Source: three-view drawing plus pictorial views. Frame: mm from the lowest corner of the part. A direction names the side the tool comes from. Give positions to 0.01 mm unless a question says otherwise; leave off trailing zeros. Order: outer loops, then holes, each group sorted by start corner. A loop starts at its lowest first (then second) coordinate and runs counter-clockwise, first axis right, second up.
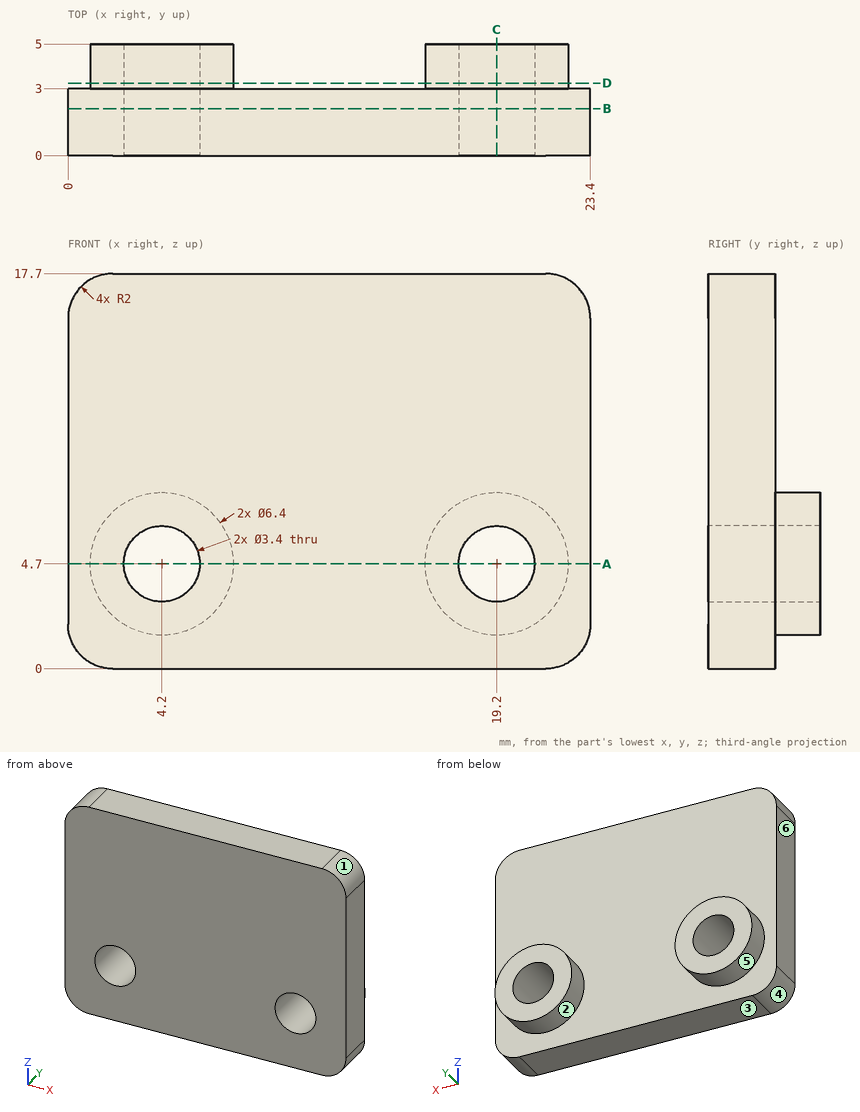
(1) Section A-A, the plane z = 4.7. Return loops of the section in (x, y), plus the area to 3 significant figures.
(2) Section B-B, the plane y = 2.1. Return loops of the section in (x, z).
(3) Section C-C, the plane x = 19.2. Return loops of the section in (y, z).
(4) Draft query along X for the marked faces 1, 2, 3 and 4. Return one class per face: +X half, -X half, draft (parallel to the pull), parting line (faces both ways), or undercut.
(5) Access query for the marked faces 5 and 6. Directions: +Z, -Z, +X, -X, +Y, -Y. A direction counts if a zero-diameter tool reaches every point of the face in a straight line with its end or side. Return the directions, or none.
(6) Line query: line 1 along X through (y, z) = (1.65, 4.7); line 2 along X through (y, z) = (4.3, 3.75); line 3 along X through (y, z) = (3.6, 4.7). Output: solid intervals per line, ascending.
(7) Section D-D, the plane y = 3.25. Return loops of the section in (x, z).
(8) Pin query (flat end, axial travel): pin 1 Ø1.5 at (x, y) = (3.5, 4.5) entering from -Z. Return the tip coordinate at first contact, or that it passes through.
Checks:
1. outline: (0, 0) - (2.5, 0) - (2.5, 5) - (1, 5) - (1, 3) - (0, 3) - close; (5.9, 0) - (17.5, 0) - (17.5, 5) - (16, 5) - (16, 3) - (7.4, 3) - (7.4, 5) - (5.9, 5) - close; (20.9, 0) - (23.4, 0) - (23.4, 3) - (22.4, 3) - (22.4, 5) - (20.9, 5) - close
1. area: 61.8 mm2
2. outline: (0, 2) arc R2 ccw to (2, 0) - (21.4, 0) arc R2 ccw to (23.4, 2) - (23.4, 15.7) arc R2 ccw to (21.4, 17.7) - (2, 17.7) arc R2 ccw to (0, 15.7) - close; hole circle Ø3.4 at (4.2, 4.7); hole circle Ø3.4 at (19.2, 4.7)
3. outline: (0, 0) - (3, 0) - (3, 1.5) - (5, 1.5) - (5, 3) - (0, 3) - close; (0, 6.4) - (5, 6.4) - (5, 7.9) - (3, 7.9) - (3, 17.7) - (0, 17.7) - close
4. face 1: +X half
4. face 2: undercut
4. face 3: draft
4. face 4: -X half
5. face 5: +Y
5. face 6: +Z, -Z, -X, +Y, -Y
6. line 1: x = 0 to 2.5, 5.9 to 17.5, 20.9 to 23.4
6. line 2: x = 1.14 to 2.79, 5.61 to 7.26, 16.14 to 17.79, 20.61 to 22.26
6. line 3: x = 1 to 2.5, 5.9 to 7.4, 16 to 17.5, 20.9 to 22.4
7. outline: circle Ø6.4 at (4.2, 4.7); circle Ø6.4 at (19.2, 4.7); hole circle Ø3.4 at (4.2, 4.7); hole circle Ø3.4 at (19.2, 4.7)
8. pin 1: stops at z = 1.5
